Part model, mm, in its own coordinate system. Face numbers are marked on the shaded views. A direction names the side the tool comes from. Coordinates: 2 decimals unless noted, no trailing zeros. Write each loop counter-clockwise with the first axis right and the second up, starting at its lowest first coordinate (ties: lowest second). Pieces come first, ordered by that corner, then holes. Notation, with made-up numbers: (28, -2.5) - (33, -2.5) arc R23 cw to (33, 21.5) - close; hole circle Ø3 at (67.5, 53.25). An arc over 180 degrees is marked (long way). Use a Markdown table: item, result.
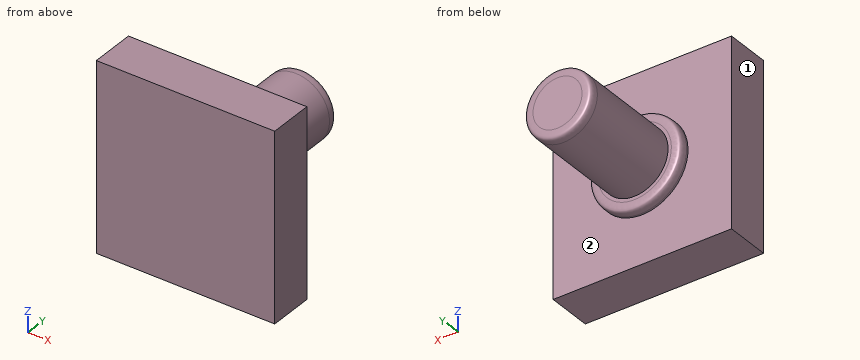
```python
from build123d import *

# Parameters (mm, degrees)
SKETCH_2_W      = 10
SKETCH_2_H      = 10.5
EXTRUDE_1_DEPTH = 2.5
SKETCH_3_R      = 2.56
EXTRUDE_2_DEPTH = 0.6
FILLET_1_SIZE   = 0.5
SKETCH_4_R      = 1.875
EXTRUDE_3_DEPTH = 6
FILLET_2_SIZE   = 0.5


with BuildPart() as part:
    # Эскиз2 → Бобышка-Вытянуть1 (new body)
    with BuildSketch(Plane(origin=(0, 0, 0), x_dir=(1, 0, 0), z_dir=(0, 1, 0))):
        Rectangle(SKETCH_2_W, SKETCH_2_H)
    extrude(amount=EXTRUDE_1_DEPTH)

    # Эскиз3 → Бобышка-Вытянуть2 (add)
    with BuildSketch(Plane(origin=(0, 2.5, 0), x_dir=(1, 0, 0), z_dir=(0, 1, 0))):
        with Locations(Location((0, 0, 0), (0, 0, 270))):
            Circle(SKETCH_3_R)
    extrude(amount=EXTRUDE_2_DEPTH)

    # Скругление1
    # a fillet whose section is not a circle: 0.5 mm, written as the material it takes off along each edge
    with BuildSketch(Plane(origin=(0, 3.1, 0), x_dir=(0, 0, 1), z_dir=(-1, 0, 0))) as fillet_1_piece_1:
        with BuildLine():
            Bezier((2.56, -FILLET_1_SIZE), (2.56, 0), (2.56 - FILLET_1_SIZE, 0), weights=[1, 2.333333333, 1])
            Line((2.56 - FILLET_1_SIZE, 0), (2.56, 0))
            Line((2.56, 0), (2.56, -FILLET_1_SIZE))
        make_face()
    revolve(axis=Axis((0, 3.1, 0), (0, 1, 0)), mode=Mode.SUBTRACT)

    # Эскиз4 → Бобышка-Вытянуть3 (add)
    with BuildSketch(Plane(origin=(0, 3.1, 0), x_dir=(1, 0, 0), z_dir=(0, 1, 0))):
        with Locations(Location((0, 0, 0), (0, 0, 270))):
            Circle(SKETCH_4_R)
    extrude(amount=EXTRUDE_3_DEPTH)

    # Скругление2
    # a fillet whose section is not a circle: 0.5 mm, written as the material it takes off along each edge
    with BuildSketch(Plane(origin=(0, 9.1, 0), x_dir=(0, 0, 1), z_dir=(-1, 0, 0))) as fillet_2_piece_1:
        with BuildLine():
            Bezier((1.875, -FILLET_2_SIZE), (1.875, 0), (1.875 - FILLET_2_SIZE, 0), weights=[1, 2.333333333, 1])
            Line((1.875 - FILLET_2_SIZE, 0), (1.875, 0))
            Line((1.875, 0), (1.875, -FILLET_2_SIZE))
        make_face()
    revolve(axis=Axis((0, 9.1, 0), (0, 1, 0)), mode=Mode.SUBTRACT)


solid = part.part
```
Item 1: Drill centre lines: probe 1 along Y at (x, z) = (3, -4.25); probe 2 along Y at (x, z) = (1.5, -1.25); probe 3 along Z at (x, y) = (0.5, 6.75). Where is each one in solid material? Low to high.
From the geometry:
| item | result |
|---|---|
| probe 1 | 0 to 2.5 |
| probe 2 | 0 to 3.1 |
| probe 3 | -1.81 to 1.81 |
Item 2: Band-saw the part on C-C, the plane x = -4. Give the cut face in (y, z).
From the geometry:
| item | result |
|---|---|
| outline | (0, -5.25) - (2.5, -5.25) - (2.5, 5.25) - (0, 5.25) - close |
Item 3: Which spindle directions (+Z, -Z, +X, -X, +Y, -Y) get a long thin tool onto all of the face, cutting with end or side? Do the marked faces 1 and 2. Say none if no direction does.
From the geometry:
| item | result |
|---|---|
| face 1 | +Z, -Z, -X, +Y, -Y |
| face 2 | +Y |
Item 4: Drop flat-ended pins along their axis: P1, Ø5, axis at y = 6.5, z = -3.5, coming from the -X side; P2, Ø1, axis at x = -3.5, z = -1.5, coming from the +Y side. Give the stop position or say it passes through.
From the geometry:
| item | result |
|---|---|
| P1 | x = -1.59 |
| P2 | y = 2.5 |
Item 5: Band-saw the part on A-A, the plane y = 6.5. Give the cut face in (x, z) (3 decimals), then the cut area to 3 significant figures.
From the geometry:
| item | result |
|---|---|
| outline | circle Ø3.75 at (0, 0) |
| area | 11.0 mm^2 |
Item 6: Band-saw the part on B-B, the plane z = 3.25. Give the cut face in (x, y).
From the geometry:
| item | result |
|---|---|
| outline | (-5, 0) - (5, 0) - (5, 2.5) - (-5, 2.5) - close |
